Read the model definition and answer for the solid it produces. Units are mm, in the model's axes. Give positions to 0.01 mm unless a question says otherwise; leave off trailing zeros. Write each loop counter-clockwise with the first axis right and the second up, starting at its lowest first coordinate (ties: lowest second). Pieces come first, ordered by that corner, then holes. Notation, with made-up numbers: (-8, 19.25) -> (25, 19.25) arc R11 ccw to (25, 39.25) -> close; hole circle Ø9 at (61.25, 82.25). An arc over 180 degrees is marked (long way). Write item = value, one per line.
Autodesk Inventor part; units mm, degrees
ref_plane "YZ Plane" through (0, 0, 0) normal (1, 0, 0) x (0, 1, 0)
ref_plane "XZ Plane" through (0, 0, 0) normal (0, 1, 0) x (-1, 0, 0)
ref_plane "XY Plane" through (0, 0, 0) normal (0, 0, 1) x (1, 0, 0)
sketch "Sketch1" plane through (0, 0, 0) normal (0, 1, 0) x (-1, 0, 0)
  line L0 (0, 0) -> (300, 0)
  line L1 (300, 0) -> (300, -300)
  line L2 (300, -300) -> (0, -300)
  line L3 (0, -300) -> (0, 0)
  dimension "d0" = 300
  dimension "d1" = 300
extrude "Extrusion1" add sketch "Sketch1" along normal blind 10
sketch "Sketch2" plane through (0, 10, 0) normal (0, 1, 0) x (1, 0, 0)
  line L0 (-300, 0) -> (0, 0)
  line L1 (0, 0) -> (0, 300)
  point P0 (-20, 20)
  point P1 (-20, 280)
  point P2 (-280, 20)
  point P3 (-280, 280)
  dimension "d4" = 20
  dimension "d5" = 20
  dimension "d8" = 260
  dimension "d11" = 260
hole "Hole1" at (-20, 10, -20) at (-20, 10, -280) at (-280, 10, -20) at (-280, 10, -280) direction (0, -1, 0) diameter 8 end through all
properties part number "Plate"
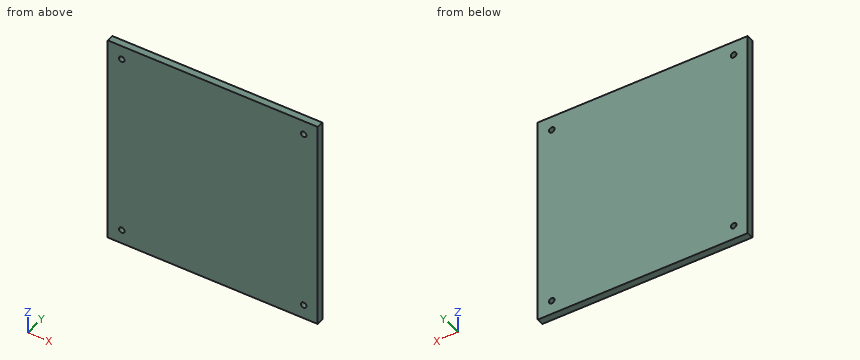
(1) The part is cut by section B-B on x = -20. Determine the outline of the cut face in (y, z).
Checks:
outline = (0, -300) -> (10, -300) -> (10, -284) -> (0, -284) -> close; (0, -276) -> (10, -276) -> (10, -24) -> (0, -24) -> close; (0, -16) -> (10, -16) -> (10, 0) -> (0, 0) -> close
(2) Given P1, Ø5, axis at x = -20, z = -280, coming from the +Y side, flat-ended and moving along its own axis, determine where the tip first touches the part or whether it passes through.
Checks:
P1 = through
(3) Consider L1, parallel to Z at x = -20, y = 4; L2, parallel to Z at x = -23, y = 3.5. Determine where each line is inside the solid, lowest interval first.
Checks:
L1 = -300 to -284, -276 to -24, -16 to 0
L2 = -300 to -282.65, -277.35 to -22.65, -17.35 to 0
(4) The part is cut by section A-A on z = -20. Determine the outline of the cut face in (x, y).
Checks:
outline = (-300, 0) -> (-284, 0) -> (-284, 10) -> (-300, 10) -> close; (-276, 0) -> (-24, 0) -> (-24, 10) -> (-276, 10) -> close; (-16, 0) -> (0, 0) -> (0, 10) -> (-16, 10) -> close
